from build123d import *

# Parameters (mm, degrees)
REVOLUTION_ANGLE            = -90
PAD_DEPTH                   = 27.85
PAD001_DEPTH                = 17.85
PAD001_MIRRORED_2_DEPTH     = 17.85
PAD_MIRRORED_2_DEPTH        = 27.85
REVOLUTION_MIRRORED_2_ANGLE = 90


with BuildPart() as part:
    # Sketch → Revolution (revolve)
    with BuildSketch(Plane.XZ):
        with BuildLine():
            Line((0, 0), (0, 5.15))
            ThreePointArc((2.15, 3), (1.52028, 4.52028), (0, 5.15))
            Line((2.15, 3), (1.075, 3))
            Line((1.075, 3), (1.075, 0))
            Line((1.075, 0), (0, 0))
        make_face()
    revolution = revolve(axis=Axis((0, 0, 0), (0, 0, 1)), revolution_arc=REVOLUTION_ANGLE)

    # Revolution Face6 → Pad (new)
    with BuildSketch(Plane(origin=(0, -0.736084, 2.777594), x_dir=(0, 1, 0), z_dir=(-1, 0, 0))):
        with BuildLine():
            Line((0.736084, -2.372406), (0.736084, 2.777594))
            Line((0.736084, 2.777594), (-0.338916, 2.777594))
            Line((-0.338916, 2.777594), (-0.338916, -0.222406))
            Line((-0.338916, -0.222406), (-1.413916, -0.222406))
            ThreePointArc((-1.413916, -0.222406), (-0.784195, -1.742686), (0.736084, -2.372406))
        make_face()
    pad = extrude(amount=PAD_DEPTH)

    # Pad Face7 → Pad001 (add)
    with BuildSketch(Plane(origin=(-13.256201, 0, 2.584242), x_dir=(1, 0, 0), z_dir=(0, 1, 0))):
        with BuildLine():
            ThreePointArc((13.256201, -2.565758), (14.776481, -1.936038), (15.406201, -0.415758))
            Line((15.406201, -0.415758), (14.331201, -0.415758))
            Line((14.331201, -0.415758), (14.331201, 2.584242))
            Line((14.331201, 2.584242), (-14.593799, 2.584242))
            Line((-14.593799, 2.584242), (-14.593799, -2.565758))
            Line((-14.593799, -2.565758), (13.256201, -2.565758))
        make_face()
    pad001 = extrude(amount=PAD001_DEPTH)

    # Pad Face7 Mirrored 2 → Pad001 Mirrored 2 (add)
    with BuildSketch(Plane(origin=(-42.443799, 0, 2.584242), x_dir=(-1, 0, 0), z_dir=(0, -1, 0))):
        with BuildLine():
            ThreePointArc((13.256201, -2.565758), (14.776481, -1.936038), (15.406201, -0.415758))
            Line((15.406201, -0.415758), (14.331201, -0.415758))
            Line((14.331201, -0.415758), (14.331201, 2.584242))
            Line((14.331201, 2.584242), (-14.593799, 2.584242))
            Line((-14.593799, 2.584242), (-14.593799, -2.565758))
            Line((-14.593799, -2.565758), (13.256201, -2.565758))
        make_face()
    pad001_mirrored_2 = extrude(amount=-PAD001_MIRRORED_2_DEPTH)

    # Revolution Face6 Mirrored 2 → Pad Mirrored 2 (add)
    with BuildSketch(Plane(origin=(-55.7, -0.736084, 2.777594), x_dir=(0, 1, 0), z_dir=(-1, 0, 0))):
        with BuildLine():
            Line((0.736084, -2.372406), (0.736084, 2.777594))
            Line((0.736084, 2.777594), (-0.338916, 2.777594))
            Line((-0.338916, 2.777594), (-0.338916, -0.222406))
            Line((-0.338916, -0.222406), (-1.413916, -0.222406))
            ThreePointArc((-1.413916, -0.222406), (-0.784195, -1.742686), (0.736084, -2.372406))
        make_face()
    pad_mirrored_2 = extrude(amount=-PAD_MIRRORED_2_DEPTH)

    # Sketch Mirrored 2 → Revolution Mirrored 2 (revolve)
    with BuildSketch(Plane(origin=(-55.7, 0, 0), x_dir=(-1, 0, 0), z_dir=(0, 1, 0))):
        with BuildLine():
            Line((0, 0), (0, 5.15))
            ThreePointArc((2.15, 3), (1.52028, 4.52028), (0, 5.15))
            Line((2.15, 3), (1.075, 3))
            Line((1.075, 3), (1.075, 0))
            Line((1.075, 0), (0, 0))
        make_face()
    revolution_mirrored_2 = revolve(axis=Axis((-55.7, 0, 0), (0, 0, 1)), revolution_arc=REVOLUTION_MIRRORED_2_ANGLE)

    # Mirrored001: Pad001, Pad, Revolution, Pad001 Mirrored 2, Pad Mirrored 2, Revolution Mirrored 2 across face of Pad001
    add(pad001.mirror(Plane(origin=(-13.256201, 17.85, 2.584242), x_dir=(-1, 0, 0), z_dir=(0, 1, 0))))
    add(pad.mirror(Plane(origin=(-13.256201, 17.85, 2.584242), x_dir=(-1, 0, 0), z_dir=(0, 1, 0))))
    add(revolution.mirror(Plane(origin=(-13.256201, 17.85, 2.584242), x_dir=(-1, 0, 0), z_dir=(0, 1, 0))))
    add(pad001_mirrored_2.mirror(Plane(origin=(-13.256201, 17.85, 2.584242), x_dir=(-1, 0, 0), z_dir=(0, 1, 0))))
    add(pad_mirrored_2.mirror(Plane(origin=(-13.256201, 17.85, 2.584242), x_dir=(-1, 0, 0), z_dir=(0, 1, 0))))
    add(revolution_mirrored_2.mirror(Plane(origin=(-13.256201, 17.85, 2.584242), x_dir=(-1, 0, 0), z_dir=(0, 1, 0))))


solid = part.part
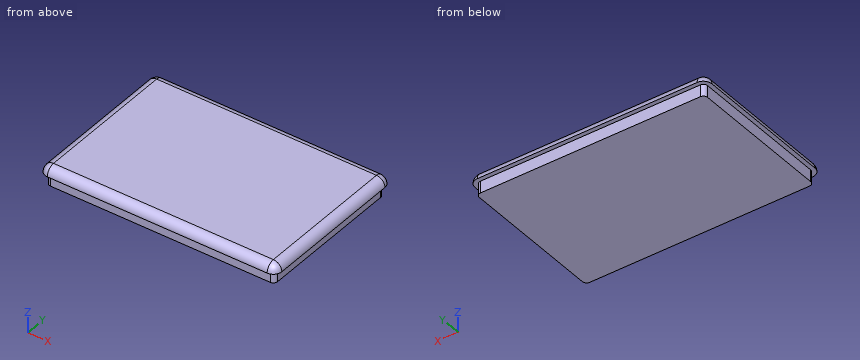
Part model, mm, in its own coordinate system. Give positions to 0.01 mm unless a question says otherwise; leave off trailing zeros. Order: outer loops, then holes, each group sorted by start corner. A loop starts at its lowest first (then second) coordinate and runs counter-clockwise, first axis right, second up. Notation, with made-up numbers: (74.5, 12) -> (99.5, 12) arc R28 ccw to (99.5, 35) -> close; hole circle Ø6 at (6.5, 81.25). An arc over 180 degrees is marked (long way). Use one line per item in the form item = value.
(1) Drill centre lines: line 1 (X direction, y = 1, z = 1.7) (3 decimals); line 2 (Y direction, x = -26.5, z = 0.9) (3 decimals); line 3 (Y direction, x = -36, z = 3.6). Where is each one in solid material? Low to high. Write a range as from..to.
Solution:
line_1 = -56.775..1.075
line_2 = -1.075..36.775
line_3 = -2.06..37.76
(2) Saw through at B-B (x = -7). Write the cut outline in (y, z) (3 decimals), then the cut area to 3 significant figures.
Solution:
outline = (-2.15, 3) -> (-1.075, 3) -> (-1.075, 0) -> (36.775, 0) -> (36.775, 3) -> (37.85, 3) arc R2.15 ccw to (35.7, 5.15) -> (0, 5.15) arc R2.15 ccw to start
area = 198 mm²
(3) Saw through at A-A (z = 1.05). Write the cut outline in (x, y) (3 decimals).
Solution:
outline = (-56.775, 0) arc R1.075 ccw to (-55.7, -1.075) -> (0, -1.075) arc R1.075 ccw to (1.075, 0) -> (1.075, 35.7) arc R1.075 ccw to (0, 36.775) -> (-55.7, 36.775) arc R1.075 ccw to (-56.775, 35.7) -> close
(4) Flat gauge pins, fed straight in: P1, Ø0.6, axis at y = -0.5, z = 4, coming from the +X side; P2, Ø2.5, axis at y = -1.5, z = 4.5, coming from the -X side; P3, Ø5, axis at x = -44, y = 21.5, coming from the -Z side; P4, Ø2.5, axis at x = -40.5, z = 1.5, coming from the +Y side (3 decimals). Where does each tip first touch, or does it go through?
Solution:
P1 = 1.99
P2 = -57.67
P3 = 0
P4 = 36.775
